Print and shaded views of the part. All mm, measured from the part's lowest x, y and z. A direction names the side the tool comes from. Round coordinates to 2 decimals unless told otherwise and drop trailing zeros. Order: outer loops, then holes, each group sorted by start corner. A loop starts at its lowest first (then second) coordinate and runs counter-clockwise, first axis right, second up. Notation, with made-up numbers: M 28,-30.75 L 51,-30.75 A33 ccw 51,4.25 Z; hole C 70,-35 d5. An arc over 180 degrees is marked long. Use CSV: the item, a comma, the result in double quotes.
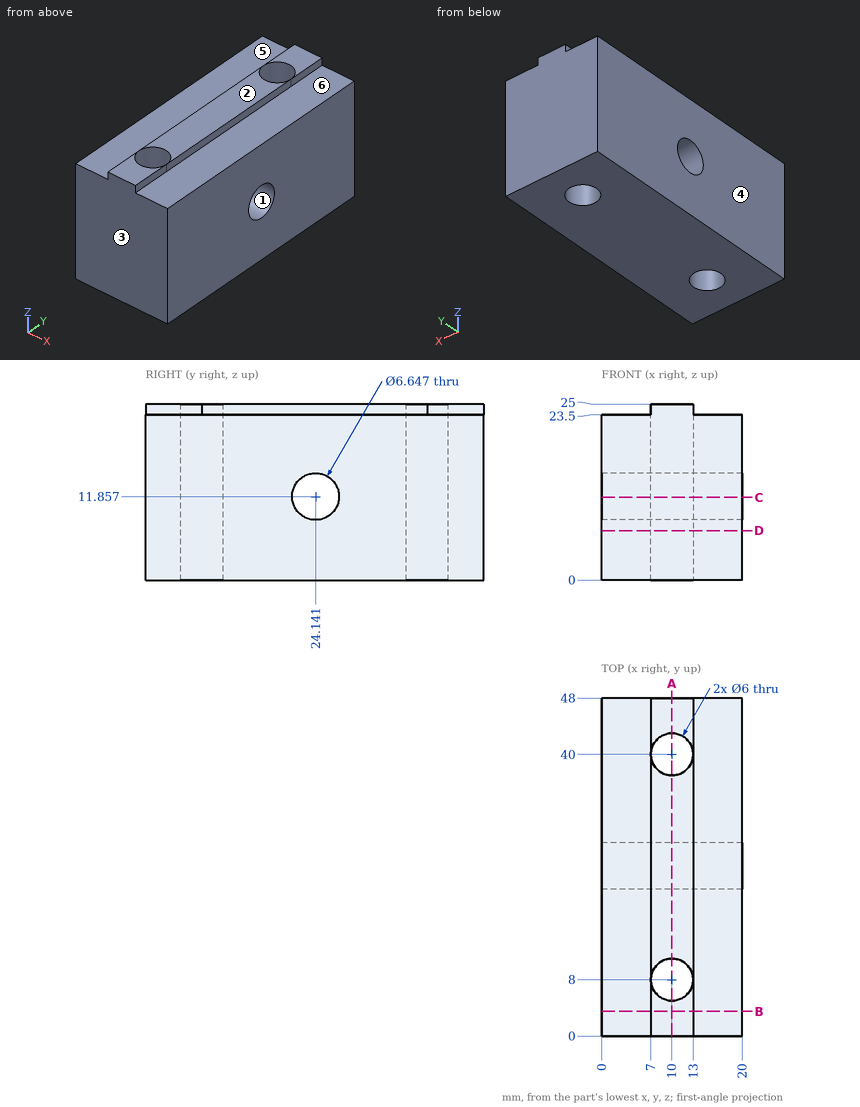
(1) Two-plate mould, pull along Z, no slides. Class the marked faces 1, 2 and 3: released by +Z, released by -Z, zero draft, split by the parting line, or undercut.
Answer block:
face 1,"undercut"
face 2,"released by +Z"
face 3,"zero draft"
(2) Drop flat-ended pins along their axis: pin 1 (2 mm diameter, centred on x = 2, y = 16, fed in from +Z); pin 2 (6 mm diameter, centred on y = 24.14, z = 11.86, fed in from +X). Give the stop position or say it passes through.
Answer block:
pin 1,"stops at z = 23.5"
pin 2,"passes through"
(3) Cut at C-C, the plane z = 11.75. Give the cut face in (x, y).
Answer block:
outline,"M 0,0 L 20,0 L 20,20.82 L 0,20.82 Z; M 0,27.46 L 20,27.46 L 20,48 L 0,48 Z; hole C 10,8 d6; hole C 10,40 d6"
(4) Tool access for the marked faces 4, 5 and 6: list every direction of +Z, -Z, +X, -X, +Y, -Y with a clear straight run to the whole face (end or side of a thin tool).
Answer block:
face 4,"+Z, -Z, -X, +Y, -Y"
face 5,"+Z, -X, +Y, -Y"
face 6,"+Z, +X, +Y, -Y"
(5) Cut at B-B, the plane y = 3.5. Give the cut face in (x, z).
Answer block:
outline,"M 0,0 L 20,0 L 20,23.5 L 13,23.5 L 13,25 L 7,25 L 7,23.5 L 0,23.5 Z"
(6) Cut at A-A, the plane x = 10. Give the cut face in (y, z).
Answer block:
outline,"M 0,0 L 5,0 L 5,25 L 0,25 Z; M 11,0 L 37,0 L 37,25 L 11,25 Z; M 43,0 L 48,0 L 48,25 L 43,25 Z; hole C 24.14,11.86 d6.65"
(7) Wall check: line 1 (Y direction, x = 10, z = 15.75); line 2 (Y direction, x = 12.5, z = 23.5); line 3 (X direction, y = 40, z = 7). Give the ranges that are in metal, low to high. Write a range as from..to.
Answer block:
line 1,"y = 0..5, 11..37, 43..48"
line 2,"y = 0..6.34, 9.66..38.34, 41.66..48"
line 3,"x = 0..7, 13..20"
(8) Cut at D-D, the plane z = 7. Give the cut face in (x, y).
Answer block:
outline,"M 0,0 L 20,0 L 20,48 L 0,48 Z; hole C 10,8 d6; hole C 10,40 d6"
